Design review of the part built by this model. Coordinates are the model's own, in mm. A direction names the side the tool comes from. Give positions to 0.01 mm unless a question says otherwise; leave off trailing zeros. Loops run counter-clockwise (first coordinate to the right, second up) from the corner with the lowest first, then second, coordinate; pieces in that order, holes last. Notation, with made-up numbers: (32.5, -36) - (59.5, -36) arc R13 ccw to (59.5, -27) - close; hole circle Ø6 at (17.25, 44.25). An arc over 180 degrees is marked (long way). Write each question's results on one line, items separated by ' | '.
```python
from build123d import *

# Parameters (mm, degrees)
SKETCH1_R               = 9.779
SKETCH1_R_2             = 5.7785
BOSS_EXTRUDE1_DEPTH     = 105.41
SKETCH2_R               = 1.905
CUT_EXTRUDE1_DEPTH      = 10.779
CUT_EXTRUDE1_DEPTH_BACK = 10.779
SKETCH3_R               = 2.54
CUT_EXTRUDE2_DEPTH      = 10.7790001
CUT_EXTRUDE2_DEPTH_BACK = 10.7790001
SKETCH4_R               = 6.604
CUT_EXTRUDE3_DEPTH      = 77.216


with BuildPart() as part:
    # Sketch1 → Boss-Extrude1 (new body)
    with BuildSketch(Plane(origin=(0, 0, 0), x_dir=(1, 0, 0), z_dir=(0, 1, 0))):
        Circle(SKETCH1_R)
        Circle(SKETCH1_R_2, mode=Mode.SUBTRACT)
    extrude(amount=BOSS_EXTRUDE1_DEPTH)

    # Sketch2 → Cut-Extrude1 (cut, two sides)
    with BuildSketch(Plane.XY) as cut_extrude1_sk:
        with Locations((0, 89.916)):
            Circle(SKETCH2_R)
    extrude(amount=CUT_EXTRUDE1_DEPTH, mode=Mode.SUBTRACT)
    extrude(cut_extrude1_sk.sketch, amount=-CUT_EXTRUDE1_DEPTH_BACK, mode=Mode.SUBTRACT)

    # Sketch3 → Cut-Extrude2 (cut, two sides)
    with BuildSketch(Plane(origin=(0, 0, 0), x_dir=(0, 0, -1), z_dir=(1, 0, 0))) as cut_extrude2_sk:
        with Locations((0, 12.7)):
            Circle(SKETCH3_R)
    extrude(amount=CUT_EXTRUDE2_DEPTH, mode=Mode.SUBTRACT)
    extrude(cut_extrude2_sk.sketch, amount=-CUT_EXTRUDE2_DEPTH_BACK, mode=Mode.SUBTRACT)

    # Sketch4 → Cut-Extrude3 (cut)
    with BuildSketch(Plane.XZ):
        Circle(SKETCH4_R)
    extrude(amount=-CUT_EXTRUDE3_DEPTH, mode=Mode.SUBTRACT)


solid = part.part
```
Item 1: Tool access review of faces 4 (the face through (5.51, 91.12, -1.74)), 5 (the face through (0, 77.216, -6)): name each direction out of +Z, -Z, +X, -X, +Y, -Y from which nothing blocks a thin tool from reaching the whole face with its end or side.
Output values:
face 4: +Y, -Y | face 5: -Y
Item 2: Clearance check with flat-ended pins moving along their axes: P1, Ø5, axis at y = 81.5, z = 4.5, coming from the +X side; P2, Ø2, axis at y = 37, z = 6, coming from the +X side; P3, Ø1, axis at x = 3, y = 76, coming from the +Z side. State where each tip first meets the part, or that it passes through.
Output values:
P1: stops at x = 9.57 | P2: stops at x = 8.4 | P3: stops at z = 9.45
Item 3: We need section D-D on y = 68.5. Give the boundary of the cut face in (x, z).
Output values:
outline: circle Ø19.56 at (0, 0); hole circle Ø13.21 at (0, 0)
Item 4: We need section A-A on x = 0. Give the boundary of the cut face in (y, z), then the cut area to 3 significant figures.
Output values:
outline: (0, -9.78) - (88.01, -9.78) - (88.01, -5.78) - (77.22, -5.78) - (77.22, -6.6) - (0, -6.6) - close; (0, 6.6) - (77.22, 6.6) - (77.22, 5.78) - (88.01, 5.78) - (88.01, 9.78) - (0, 9.78) - close; (91.82, -9.78) - (105.41, -9.78) - (105.41, -5.78) - (91.82, -5.78) - close; (91.82, 5.78) - (105.41, 5.78) - (105.41, 9.78) - (91.82, 9.78) - close | area: 685 mm²
Item 5: Wall thickness on probe 1 along Z at (x, y) = (0, 37); probe 2 along Y at (x, z) = (-8.6, 0); probe 3 along X at (y, z) = (35, -0.5): over which ranges is each line inside the solid? List them lowest first.
Output values:
probe 1: z = -9.78 to -6.6, 6.6 to 9.78 | probe 2: y = 0 to 10.16, 15.24 to 105.41 | probe 3: x = -9.77 to -6.59, 6.59 to 9.77
Item 6: We need section B-B on z = 0. Give the boundary of the cut face in (x, y), then the cut area to 3 significant figures.
Output values:
outline: (-9.78, 0) - (-6.6, 0) - (-6.6, 10.16) - (-9.78, 10.16) - close; (-9.78, 15.24) - (-6.6, 15.24) - (-6.6, 77.22) - (-5.78, 77.22) - (-5.78, 105.41) - (-9.78, 105.41) - close; (5.78, 77.22) - (6.6, 77.22) - (6.6, 15.24) - (9.78, 15.24) - (9.78, 105.41) - (5.78, 105.41) - close; (6.6, 0) - (9.78, 0) - (9.78, 10.16) - (6.6, 10.16) - close | area: 684 mm²
Item 7: We need section C-C on x = 4.5. Give the boundary of the cut face in (y, z).
Output values:
outline: (0, -8.68) - (105.41, -8.68) - (105.41, -3.63) - (77.22, -3.63) - (77.22, -4.83) - (0, -4.83) - close; (0, 4.83) - (77.22, 4.83) - (77.22, 3.63) - (105.41, 3.63) - (105.41, 8.68) - (0, 8.68) - close
Item 8: Draft analysis for pull direction Z (two halves, no side actions). For faces 1 (the face through (6.4, 0, -2.3)), 2 (the face through (-7.91, 15.22, 0.33)), 3 (the face through (-2.12, 51.967, 9.546)), state which applies: +Z half, -Z half, draft (parallel to the pull), parting line (faces both ways), or undercut.
Output values:
face 1: draft | face 2: undercut | face 3: parting line
